from build123d import *

# Parameters (mm, degrees)
SKETCH_R      = 5
PAD_DEPTH     = 5
SKETCH001_R   = 5
SKETCH001_R_2 = 1.7
PAD001_DEPTH  = 1


with BuildPart() as part:
    # Sketch → Pad (new body)
    with BuildSketch(Plane.XY):
        Circle(SKETCH_R)
        Polygon((-3.290897, 0), (-1.645448, -2.85), (1.645448, -2.85), (3.290897, 0), (1.645448, 2.85), (-1.645448, 2.85), align=None, mode=Mode.SUBTRACT)
    extrude(amount=PAD_DEPTH)

    # Sketch001 → Pad001 (join)
    with BuildSketch(Plane.XY):
        Circle(SKETCH001_R)
        Circle(SKETCH001_R_2, mode=Mode.SUBTRACT)
    extrude(amount=PAD001_DEPTH)


solid = part.part
Work out the finished part from the listing and answer in its coordinate system (mm). A direction names the side the tool comes from. Round coordinates to 2 decimals unless told otherwise and drop trailing zeros. Write each loop counter-clockwise with the first axis right and the second up, starting at its lowest first coordinate (ties: lowest second). Pieces come first, ordered by that corner, then holes. Notation, with made-up numbers: M -31,-39 L -22,-39 A23 cw -22,-20 Z; hole C 26.5,-21 d3. An arc over 180 degrees is marked long. Use a Markdown table: item, result.
1) The part is cut by section B-B on z = 2.1. Give the vertices of the cut face in (x, y), plus the area to 3 significant figures.
Taken from the geometry:
| item | result |
|---|---|
| outline | C 0,0 d10; hole M -3.29,0 L -1.65,-2.85 L 1.65,-2.85 L 3.29,0 L 1.65,2.85 L -1.65,2.85 Z |
| area | 50.4 mm2 |
2) Which of the six approach directions +Z, -Z, +X, -X, +Y, -Y give full straight-line access (tool end or side, diameter ignored) to faces 4 (the face through (1.4, 1.3, 1)), 5 (the face through (0, -2, 0))?
Taken from the geometry:
| item | result |
|---|---|
| face 4 | +Z |
| face 5 | -Z, +X, -X, +Y, -Y |
3) The part is cut by section A-A on x = 0. Give the vertices of the cut face in (y, z), plus the area to 3 significant figures.
Taken from the geometry:
| item | result |
|---|---|
| outline | M -5,0 L -1.7,0 L -1.7,1 L -2.85,1 L -2.85,5 L -5,5 Z; M 1.7,0 L 5,0 L 5,5 L 2.85,5 L 2.85,1 L 1.7,1 Z |
| area | 23.8 mm2 |
4) The part is cut by section D-D on x = -2. Give the vertices of the cut face in (y, z), plus the area to 3 significant figures.
Taken from the geometry:
| item | result |
|---|---|
| outline | M -4.58,0 L 4.58,0 L 4.58,5 L 2.24,5 L 2.24,1 L -2.24,1 L -2.24,5 L -4.58,5 Z |
| area | 27.9 mm2 |
5) Flat-ended cylindrical pins translate along their axes: pin 1 (2 mm diameter, centred on x = -1.5, z = 4, fed in from -Y); pin 2 (1.7 mm diameter, centred on x = 0, y = -1, fed in from +Z); pin 3 (1 mm diameter, centred on x = -0.5, z = 2, fed in from +Y); pin 4 (2 mm diameter, centred on y = -1.5, z = 2, fed in from +X). Find the tip coordinate at first contact, or state that the pin passes through.
Taken from the geometry:
| item | result |
|---|---|
| pin 1 | stops at y = -4.97 |
| pin 2 | stops at z = 1 |
| pin 3 | stops at y = 5 |
| pin 4 | stops at x = 4.97 |
6) Determine the mould class of faces 1 (the face through (2.2, -2.2, 5)), 2 (the face through (2.48, 1.405, 2.972)), 3 (the face through (-1.08, -4.88, 2.46)) for opening direction Y: pulls with the +Y half, pulls with the -Y half, needs draft (parallel to the pull), parting line crosses it, or undercut.
Taken from the geometry:
| item | result |
|---|---|
| face 1 | needs draft |
| face 2 | undercut |
| face 3 | parting line crosses it |
7) The part is cut by section C-C on y = -0.75. Give the vertices of the cut face in (x, z), plus the area to 3 significant figures.
Taken from the geometry:
| item | result |
|---|---|
| outline | M -4.94,0 L -1.53,0 L -1.53,1 L -2.86,1 L -2.86,5 L -4.94,5 Z; M 1.53,0 L 4.94,0 L 4.94,5 L 2.86,5 L 2.86,1 L 1.53,1 Z |
| area | 23.5 mm2 |
8) Consider line 1 (Y direction, x = 0, z = 0.7); line 2 (Y direction, x = 0, z = 2.4); line 3 (Z direction, x = 1, y = -2.5). Determine where each line is inside the solid, lowest interval first. Write a range as [from, to].
Taken from the geometry:
| item | result |
|---|---|
| line 1 | y = [-5, -1.7], [1.7, 5] |
| line 2 | y = [-5, -2.85], [2.85, 5] |
| line 3 | z = [0, 1] |
